Autodesk Inventor part; units mm, degrees
ref_plane "IDS_WORKPLANE{1}" through (-6.4262, 0, 0) normal (1, 0, 0) x (0, 0, -1)
ref_plane "Work Plane2" through (41.275, 0, 0) normal (0, 0, -1) x (1, 0, 0)
ref_plane "YZ Plane" through (0, 0, 0) normal (1, 0, 0) x (0, 1, 0)
sketch "Szkic1" plane through (0, 0, 0) normal (0, 0, 1) x (1, 0, 0)
  line L0 (-6.4262, 0) -> (12.7, 0)
  line L1 (12.7, 0) -> (12.7, 3.9687)
  line L2 (12.7, 3.9687) -> (3.5281, 3.9687)
  line L3 (3.5281, 3.9687) -> (2.6812, 3.9688)
  line L4 (2.6812, 3.9688) -> (0, 3.9688)
  line L5 (0, 3.9688) -> (0, 5.5499)
  line L6 (-10.6898, 0) -> (16.5983, 0)
  line L7 (0, -1.1296) -> (0, 6.7773)
  line L8 (0, 5.5499) -> (-4.9391, 5.5499)
  arc A0 (-4.9391, 5.5499) -> (-6.4262, 0) centre (4.6736, 0) ccw
  line L9 (3.5281, 3.9687) -> (0, 3.9687) construction
  dimension "d0" = 12.7
  dimension "d1" = 9.1719
  dimension "d2" = 0.8468
  dimension "d3" = 6.4262
  dimension "d4" = 7.9375
  dimension "d5" = 7.9375
  dimension "d9" = 11.0998
  dimension "d10" = 0
  dimension "d13" = 11.0998
revolve "Bryła" add sketch "Szkic1" angle 360 about axis through (-6.4262, 0, 0) along (1, 0, 0)
ref_plane "IDS_WORKPLANE{1}" through (-6.4262, 0, 0) normal (1, 0, 0) x (0, 0, -1)
sketch "Szkic2" plane through (-6.4262, 0, 0) normal (1, 0, 0) x (0, 0, -1)
  circle A0 centre (0, 0) radius 5.5499
  line L0 (0, -7.7699) -> (0, 7.7699)
  line L1 (7.7699, 0) -> (-7.7699, 0)
  line L2 (-5.5499, 1.0668) -> (5.5499, 1.0668)
  line L3 (5.5499, 1.0668) -> (5.5499, -1.0668)
  line L4 (5.5499, -1.0668) -> (-5.5499, -1.0668)
  line L5 (-5.5499, -1.0668) -> (-5.5499, 1.0668)
  line L6 (-5.5499, 0) -> (5.5499, 0) construction
  line L7 (0, 1.0668) -> (0, -1.0668) construction
  dimension "d15" = 2.1336
extrude "Szczelina" cut sketch "Szkic2" along normal blind 2.921 contours L1 L0 L2 A0 | L3 L4 A0 | A0 L4 L0 L1 | A0 L2 L3 | L1 A0 L2 L0 | L0 L4 A0 L1 | L5 L2 A0 | A0 L4 L5
thread "Gwint"
sketch "Szkic3" plane through (0, 0, 0) normal (0, 0, 1) x (1, 0, 0)
  line L0 (12.7, 0) -> (12.7, 3.9687)
  line L1 (12.7, 3.9687) -> (3.5281, 3.9687)
  line L2 (-6.4262, 0) -> (12.7, 0)
  arc A0 (12.7, 0) -> (11.6366, 3.9687) centre (4.7625, 0) ccw
  line L3 (12.7, -3.9687) -> (12.7, 3.9687)
  line L4 (11.6366, 3.9687) -> (11.6366, 0)
  line L5 (11.6366, 0) -> (12.7, 0)
  dimension "d40" = 7.9375
revolve "Zaokrąglenie1" cut sketch "Szkic3" angle 360 about axis through (-6.4262, 0, 0) along (1, 0, 0) contours A0 L1 L0
chamfer "Faza" distance 0.7056 angle 45 1 edges at (11.6366, -3.9687, 0)
ref_plane "Work Plane2" through (41.275, 0, 0) normal (0, 0, -1) x (1, 0, 0)
fillet "Zaokrąglenie4" radius 0.7874 1 edges at (0, -3.9688, 0)
equation "\"d0\" = NLG"
equation "\"d1\" = GEL"
equation "\"d2\" = GAL"
equation "\"d3\" = KOH"
equation "\"d4\" = GD"
equation "\"d5\" = BDM"
equation "\"d9\" = KOD"
equation "\"d13\" = KR"
equation "\"d15\" = SBR"
equation "\"d16\" = STI"
equation "\"d40\" = GD"
equation "\"d11\" = GEL"
equation "\"d43\" = 0.5 * RR"
equation "\"d46\" = R"
equation "\"GD\" = NND"
equation "\"NLG\" = 12.7"
equation "\"GEL\" = 9.17194"
equation "\"KOD\" = 11.0998"
equation "\"KOH\" = 6.4262"
equation "\"GAL\" = 0.84684"
equation "\"BDM\" = NND"
equation "\"SBR\" = 2.1336"
equation "\"STI\" = 2.921"
equation "\"KEWI\" = 0"
equation "\"KR\" = KOD"
equation "\"d14\" = -KOH"
equation "\"R\" = 0.7874"
equation "\"THREADDIA\" = 7.9375"
equation "\"TOA\" = 30deg"
equation "\"KOH1\" = 5.1562"
equation "\"NND\" = 7.9375"
equation "\"GD1\" = 6.25856"
equation "\"THREADDESC\" = 1.2345"
properties part number "ANSI B18.6.2 - 5/16-18 UNC - 0,5" material "Stal, miękka"
Design review of the part built by this model. Coordinates are the model's own, in mm. A direction names the side the tool comes from. Coordinates: 2 decimals unless noted, no trailing zeros. Loops run counter-clockwise (first coordinate to the right, second up) from the corner with the lowest first, then second, coordinate; pieces in that order, holes last. Notation, with made-up numbers: (49.5, 12.25) -> (56.5, 12.25) arc R14 cw to (56.5, 32.25) -> close; hole circle Ø9 at (57, -33.75). An arc over 180 degrees is marked (long way). Use a Markdown table: item, result. Add a question column.
Item 1: Machinability: for faces 1 (the flat face through (-5, 1.067, 0)), 2 (the cylindrical face through (1.721, 3.666, 1.52)), 3 (the cylindrical face through (-2.504, 2.561, 4.924)), which of the approach directions +Z, -Z, +X, -X, +Y, -Y give a long, thin tool a straight path to every point of the face, cutting with its end or side? Answer none if there is none.
Item 2: Wall thickness on L1, parallel to Z at x = 9.75, y = 0; L2, parallel to Z at x = -5, y = -1.5; L3, parallel to X at y = 1.25, z = -2.75: over which ranges is each line inside the solid? List them lowest first. Write a range as from..to.
Item 3: Clearance check with flat-ended pins moving along their axes: P1, Ø0.9, axis at x = -5, z = 2.5, coming from the +Y side; P2, Ø6, axis at y = 0.5, z = 0.5, coming from the -X side; P3, Ø1, axis at y = -3.5, z = -2.5, coming from the +X side; P4, Ø4, axis at y = 1.5, z = 3, coming from the -X side. State where each tip first meets the part, or that it passes through.
Item 4: We need section A-A, the plane x = -1. Write out the cut boundary in (y, z), and give its area (3 significant figures).
Numbers:
| question | item | result |
|---|---|---|
| 1 | face 1 | +Z, -Z, -X |
| 1 | face 2 | +X |
| 1 | face 3 | +X, -X |
| 2 | L1 | z = -3.97..3.97 |
| 2 | L2 | z = -5.23..5.23 |
| 2 | L3 | x = -6.01..12.1 |
| 3 | P1 | stops at y = 5.16 |
| 3 | P2 | stops at x = -6.37 |
| 3 | P3 | stops at x = 11.21 |
| 3 | P4 | stops at x = -6.33 |
| 4 | outline | circle Ø11.1 at (0, 0) |
| 4 | area | 96.8 mm^2 |
